Verification items for this drawing (mm, ordinates from the low corner). Round coordinates to 2 decimals unless told otherwise and drop trailing zeros. Order: outer loops, then holes, each group sorted by start corner. A loop starts at its lowest first (then second) coordinate and runs counter-clockwise, first axis right, second up. Notation, with made-up numbers: (17, 88.25) -> (24, 88.25) arc R21 cw to (24, 122.25) -> close; hole circle Ø10 at (-14.75, 18.25). An arc over 180 degrees is marked (long way). Return JSON: item names as keys, results as strings. Group by question number.
Item 1: Sectioned sample at D-D on y = 56.5. Record the cut outline in (x, z), plus the area to 3 significant figures.
Item 2: Scan lines: probe 1 along X at (y, z) = (69, 2.15); probe 2 along Y at (x, z) = (98, 1.8); probe 3 along Y at (x, z) = (119.5, 1.8). Record each from-to range of solid material in increasing order. Write a range as from..to.
Item 3: Sectioned sample at A-A on z = 0.6. Record the cut outline in (x, y).
Item 4: Sectioned sample at C-C on x = 92. Record the cut outline in (y, z).
Item 5: Sectioned sample at B-B on y = 11. Record the cut outline in (x, z).
Item 6: Depth check by flat-ended pin: pin 1 Ø6 at (x, y) = (16.5, 39.5) entering from -Z. Enter the tip coordinate at first touch or a pass-through.
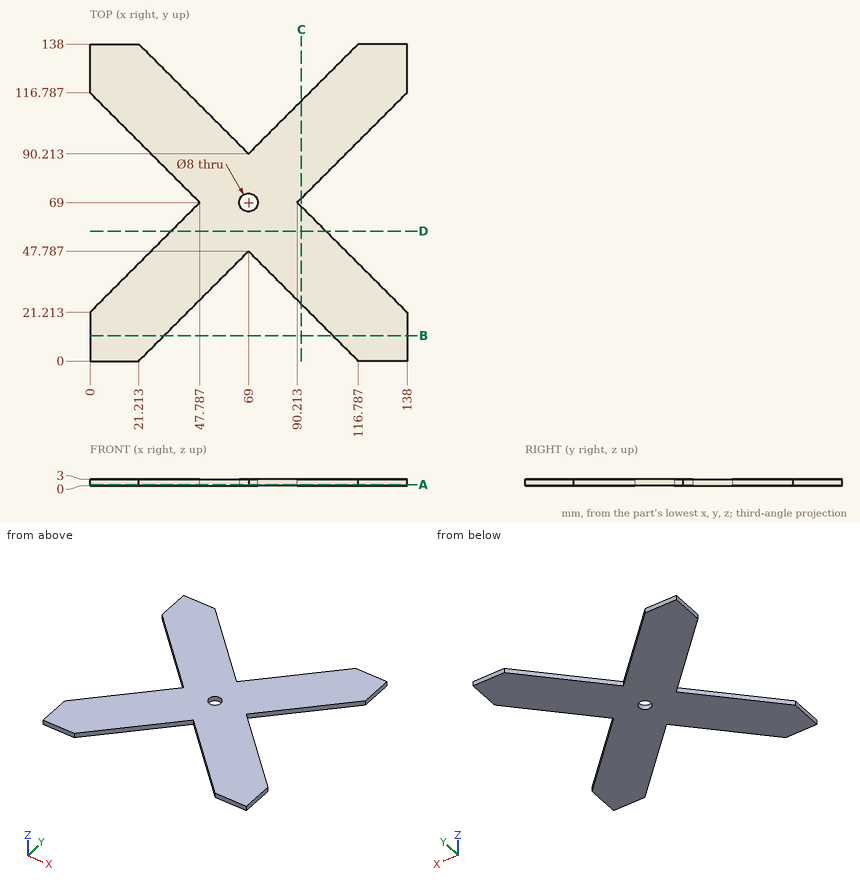
Recorded:
{
 "1": {"outline": "(35.29, 0) -> (102.71, 0) -> (102.71, 3) -> (35.29, 3) -> close", "area": "202 mm²"},
 "2": {"probe 1": "47.79..65, 73..90.21", "probe 2": "18.79..61.21, 76.79..119.21", "probe 3": "0..39.71, 98.29..138"},
 "3": {"outline": "(0, 0) -> (21.21, 0) -> (69, 47.79) -> (116.79, 0) -> (138, 0) -> (138, 21.21) -> (90.21, 69) -> (138, 116.79) -> (138, 138) -> (116.79, 138) -> (69, 90.21) -> (21.21, 138) -> (0, 138) -> (0, 116.79) -> (47.79, 69) -> (0, 21.21) -> close; hole circle Ø8 at (69, 69)"},
 "4": {"outline": "(24.79, 0) -> (67.21, 0) -> (67.21, 3) -> (24.79, 3) -> close; (70.79, 0) -> (113.21, 0) -> (113.21, 3) -> (70.79, 3) -> close"},
 "5": {"outline": "(0, 0) -> (32.21, 0) -> (32.21, 3) -> (0, 3) -> close; (105.79, 0) -> (138, 0) -> (138, 3) -> (105.79, 3) -> close"},
 "6": {"pin 1": "z = 0"}
}
